Here's how the part is built. I have some questions about the finished solid (model axes, mm). A direction names the side the tool comes from. Round coordinates to 2 decimals unless told otherwise and drop trailing zeros. Write each loop counter-clockwise with the first axis right and the second up, starting at its lowest first coordinate (ties: lowest second). Pieces come first, ordered by that corner, then holes. Notation, with made-up numbers: (-9.75, 51.25) -> (10.25, 51.25) arc R12 cw to (10.25, 68.25) -> close; hole circle Ø4 at (-20.5, 87.5). An arc over 180 degrees is marked (long way). Put each result on its own line as item: value. Start each with the question number.
1) Which directions (+Z, -Z, +X, -X, +Y, -Y) give clear straight access to the entire face, cutting with the end or side of a thin tool? Please do faces 1 (the cylindrical face through (-1.5, -2.46, 0.07)), 2 (the flat face through (0, 2, -2.35)).
2) We'd pull the mould along Z, two halves only. Please class faces 3 (the flat face through (0, 5, -2)), 4 (the flat face through (0, 1, 0)), 5 (the flat face through (-2.045, 2.465, 1.159)), 6 (the cylindrical face through (-1.27, 3.03, 0.97)): released by +Z, released by -Z, zero draft, split by the parting line, or undercut.
3) I want a section at D-D, the plane y = -2.25. List the corners of the cut face in (x, z) for me.
4) I want a section at C-C, the plane z = -1. List the corners of the cut face in (x, y) for me.
5) Will these pins go through, and if not, where does the flat tip stop? P1, Ø2, axis at x = 0, z = -0.5, coming from the +Y side; P2, Ø2, axis at y = -3.5, z = 0.5, coming from the -X side; P3, Ø1, axis at x = -2, z = 0.5, coming from the -Y side.
6) If I drill on line 1 along Z through (x, y) = (0, 2.85); line 2 along Y through (x, z) = (1.65, 1.7); line 3 along Y through (x, z) = (-1.05, -0.1), over which ranges is the centre line in solid material (lowest first)? Write a range as [from, to].
7) I want a section at A-A, the plane y = 0.5. List the corners of the cut face in (x, z) for me.
8) I want a section at B-B, the plane x = 0. List the corners of the cut face in (y, z) for me, then the cut area to 3 significant figures.
from build123d import *

# Parameters (mm, degrees)
EXTRUDE_1_DEPTH     = 5
SKETCH_2_R          = 1.6
CUT_EXTRUDE_1_DEPTH = 4
SKETCH_3_R          = 1.5
EXTRUDE_2_DEPTH     = 5


with BuildPart() as part:
    # 草图1 → 凸台-拉伸1 (new body)
    with BuildSketch(Plane(origin=(0, 0, 0), x_dir=(1, 0, 0), z_dir=(0, 1, 0))):
        Polygon((2.713546265, 0), (1.356773133, 2.35), (-1.356773133, 2.35), (-2.713546265, 0), (-1.356773133, -2.35), (1.356773133, -2.35), align=None)
    extrude(amount=EXTRUDE_1_DEPTH)

    # 草图2 → 切除-拉伸1 (cut)
    with BuildSketch(Plane(origin=(0, 5, 0), x_dir=(1, 0, 0), z_dir=(0, 1, 0))):
        Circle(SKETCH_2_R)
    extrude(amount=-CUT_EXTRUDE_1_DEPTH, mode=Mode.SUBTRACT)

    # 草图3 → 凸台-拉伸2 (add)
    with BuildSketch(Plane.XZ):
        Circle(SKETCH_3_R)
    extrude(amount=EXTRUDE_2_DEPTH)


solid = part.part
Findings:
1. face 1: -Y
1. face 2: -Z, +X, -X, +Y, -Y
2. face 3: zero draft
2. face 4: undercut
2. face 5: released by +Z
2. face 6: undercut
3. outline: circle Ø3 at (0, 0)
4. outline: (-2.14, 0) -> (-1.12, 0) -> (-1.12, -5) -> (1.12, -5) -> (1.12, 0) -> (2.14, 0) -> (2.14, 5) -> (1.25, 5) -> (1.25, 1) -> (-1.25, 1) -> (-1.25, 5) -> (-2.14, 5) -> close
5. P1: stops at y = 1
5. P2: stops at x = -1.5
5. P3: stops at y = 0
6. line 1: z = [-2.35, -1.6], [1.6, 2.35]
6. line 2: y = [0, 5]
6. line 3: y = [-5, 1]
7. outline: (-2.71, 0) -> (-1.36, -2.35) -> (1.36, -2.35) -> (2.71, 0) -> (1.36, 2.35) -> (-1.36, 2.35) -> close
8. outline: (-5, -1.5) -> (0, -1.5) -> (0, -2.35) -> (5, -2.35) -> (5, -1.6) -> (1, -1.6) -> (1, 1.6) -> (5, 1.6) -> (5, 2.35) -> (0, 2.35) -> (0, 1.5) -> (-5, 1.5) -> close
8. area: 25.7 mm2
